Read the model definition and answer for the solid it produces. Units are mm, in the model's axes. Coordinates: 2 decimals unless noted, no trailing zeros. Write each loop counter-clockwise with the first axis right and the second up, starting at its lowest first coordinate (ties: lowest second). Pieces come first, ordered by that corner, then holes. Notation, with made-up numbers: (56, 53) -> (83, 53) arc R15 ccw to (83, 77) -> close; hole circle Ø5 at (4, -27). An arc over 180 degrees is marked (long way). Write item = value, one per line. Start each with the question number.
1) Flat-ended cylindrical pins translate along their axes: pin 1 Ø5.5 at (x, z) = (37, -100) entering from +Y; pin 2 Ø14 at (x, z) = (91.59, 59.68) entering from -Y; pin 3 Ø7 at (x, z) = (-77.5, 115) entering from -Y. Find the tip coordinate at first contact, or state that the pin passes through.
2) Section A-A (x = 0) is taken. Determine the outline of the cut face in (y, z), plus the area to 3 significant figures.
3) Section B-B (y = -6.5) is taken. Count the separate pieces of the cut face and the enclosed holes in it, plus the area to 3 significant figures.
4) Section C-C (x = 77.5) is taken. Determine the outline of the cut face in (y, z), plus the area to 3 significant figures.
5) Find the intervals of material crossed by line 1 along Z through (x, y) = (0, -3.5); line 2 along Z through (x, y) = (-76.2, -9.8); line 3 along Z through (x, y) = (42.5, -3.5), in increasing order. Write a range as from..to.
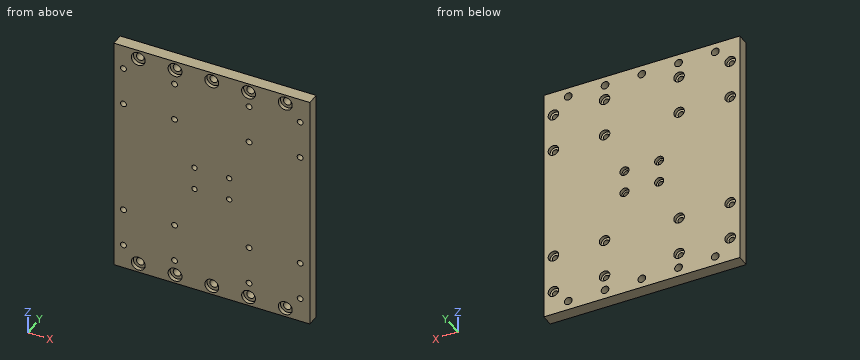
from build123d import *

# Parameters (mm, degrees)
F0_W      = 203.2
F0_H      = 249.9106
F0_R      = 3.048
F1_DEPTH  = 12.7
F2_R      = 2.794
F3_DEPTH  = 12.701
F4_R      = 4.0005
F5_DEPTH  = 12.701
F6_DEPTH  = 12.701
F7_R      = 7.1882
F8_DEPTH  = 4.064
F9_R      = 5.461
F9_R_2    = 4.699
F10_DEPTH = 3.81


with BuildPart() as f1:
    # F0 (on Front) → F1 (new body)
    with BuildSketch(Plane.XZ):
        Rectangle(F0_W, F0_H)
        with Locations((-91.5924, -99.5553)):
            Circle(F0_R, mode=Mode.SUBTRACT)
        with Locations((-38.6334, -99.5553)):
            Circle(F0_R, mode=Mode.SUBTRACT)
        with Locations((-91.5924, -59.6773)):
            Circle(F0_R, mode=Mode.SUBTRACT)
        with Locations((-38.6334, -59.6773)):
            Circle(F0_R, mode=Mode.SUBTRACT)
        with Locations((38.6334, -99.5553)):
            Circle(F0_R, mode=Mode.SUBTRACT)
        with Locations((91.5924, -99.5553)):
            Circle(F0_R, mode=Mode.SUBTRACT)
        with Locations((38.6334, -59.6773)):
            Circle(F0_R, mode=Mode.SUBTRACT)
        with Locations((91.5924, -59.6773)):
            Circle(F0_R, mode=Mode.SUBTRACT)
        with Locations((-91.5924, 59.6773)):
            Circle(F0_R, mode=Mode.SUBTRACT)
        with Locations((-38.6334, 59.6773)):
            Circle(F0_R, mode=Mode.SUBTRACT)
        with Locations((-91.5924, 99.5553)):
            Circle(F0_R, mode=Mode.SUBTRACT)
        with Locations((-38.6334, 99.5553)):
            Circle(F0_R, mode=Mode.SUBTRACT)
        with Locations((38.6334, 59.6773)):
            Circle(F0_R, mode=Mode.SUBTRACT)
        with Locations((91.5924, 59.6773)):
            Circle(F0_R, mode=Mode.SUBTRACT)
        with Locations((38.6334, 99.5553)):
            Circle(F0_R, mode=Mode.SUBTRACT)
        with Locations((91.5924, 99.5553)):
            Circle(F0_R, mode=Mode.SUBTRACT)
    extrude(amount=F1_DEPTH)

    # F2 (on face) → F3 (cut, through all)
    with BuildSketch(Plane.XZ.offset(12.7)):
        with Locations((-17.9959, 11.938)):
            Circle(F2_R)
        with Locations((17.9959, 11.938)):
            Circle(F2_R)
        with Locations((17.9959, -11.938)):
            Circle(F2_R)
        with Locations((-17.9959, -11.938)):
            Circle(F2_R)
    extrude(amount=-F3_DEPTH, mode=Mode.SUBTRACT)

    # F4 (on face) → F5 (cut, through all)
    with BuildSketch(Plane.XZ.offset(12.7)):
        with Locations((-76.2, 115.4303)):
            Circle(F4_R)
        with Locations((-38.1, 115.4303)):
            Circle(F4_R)
        with Locations((0, 115.4303)):
            Circle(F4_R)
        with Locations((38.1, 115.4303)):
            Circle(F4_R)
        with Locations((76.2, 115.4303)):
            Circle(F4_R)
        with Locations((-76.2, -115.4303)):
            Circle(F4_R)
        with Locations((-38.1, -115.4303)):
            Circle(F4_R)
        with Locations((0, -115.4303)):
            Circle(F4_R)
        with Locations((38.1, -115.4303)):
            Circle(F4_R)
        with Locations((76.2, -115.4303)):
            Circle(F4_R)
    extrude(amount=-F5_DEPTH, mode=Mode.SUBTRACT)

    # F2 (on face) → F6 (cut, through all)
    with BuildSketch(Plane.XZ.offset(12.7)):
        with Locations((-17.9959, 11.938)):
            Circle(F2_R)
        with Locations((17.9959, 11.938)):
            Circle(F2_R)
        with Locations((17.9959, -11.938)):
            Circle(F2_R)
        with Locations((-17.9959, -11.938)):
            Circle(F2_R)
    extrude(amount=-F6_DEPTH, mode=Mode.SUBTRACT)

    # F7 (on face) → F8 (cut)
    with BuildSketch(Plane.XZ.offset(12.7)):
        with Locations((0, -115.4303)):
            Circle(F7_R)
        with Locations((0, 115.4303)):
            Circle(F7_R)
        with Locations((-38.1, -115.4303)):
            Circle(F7_R)
        with Locations((-76.2, -115.4303)):
            Circle(F7_R)
        with Locations((38.1, -115.4303)):
            Circle(F7_R)
        with Locations((76.2, -115.4303)):
            Circle(F7_R)
        with Locations((-76.2, 115.4303)):
            Circle(F7_R)
        with Locations((-38.1, 115.4303)):
            Circle(F7_R)
        with Locations((38.1, 115.4303)):
            Circle(F7_R)
        with Locations((76.2, 115.4303)):
            Circle(F7_R)
    extrude(amount=-F8_DEPTH, mode=Mode.SUBTRACT)

    # F9 (on face) → F10 (cut)
    with BuildSketch(Plane(origin=(0, 0, 0), x_dir=(-1, 0, 0), z_dir=(0, 1, 0))):
        with Locations((-91.5924, 99.5553)):
            Circle(F9_R)
        with Locations((-38.6334, 99.5553)):
            Circle(F9_R)
        with Locations((38.6334, 99.5553)):
            Circle(F9_R)
        with Locations((91.5924, 99.5553)):
            Circle(F9_R)
        with Locations((-91.5924, 59.6773)):
            Circle(F9_R)
        with Locations((-38.6334, 59.6773)):
            Circle(F9_R)
        with Locations((38.6334, 59.6773)):
            Circle(F9_R)
        with Locations((91.5924, 59.6773)):
            Circle(F9_R)
        with Locations((-91.5924, -59.6773)):
            Circle(F9_R)
        with Locations((-38.6334, -59.6773)):
            Circle(F9_R)
        with Locations((38.6334, -59.6773)):
            Circle(F9_R)
        with Locations((91.5924, -59.6773)):
            Circle(F9_R)
        with Locations((91.5924, -99.5553)):
            Circle(F9_R)
        with Locations((38.6334, -99.5553)):
            Circle(F9_R)
        with Locations((-38.6334, -99.5553)):
            Circle(F9_R)
        with Locations((-91.5924, -99.5553)):
            Circle(F9_R)
        with Locations((-17.9959, 11.938)):
            Circle(F9_R_2)
        with Locations((17.9959, 11.938)):
            Circle(F9_R_2)
        with Locations((17.9959, -11.938)):
            Circle(F9_R_2)
        with Locations((-17.9959, -11.938)):
            Circle(F9_R_2)
    extrude(amount=-F10_DEPTH, mode=Mode.SUBTRACT)


solid = f1.part
Answer key:
q1.pin_1 = -3.81
q1.pin_2 = -12.7
q1.pin_3 = -8.64
q2.outline = (-12.7, -124.96) -> (0, -124.96) -> (0, -119.43) -> (-8.64, -119.43) -> (-8.64, -122.62) -> (-12.7, -122.62) -> close; (-12.7, -108.24) -> (-8.64, -108.24) -> (-8.64, -111.43) -> (0, -111.43) -> (0, 111.43) -> (-8.64, 111.43) -> (-8.64, 108.24) -> (-12.7, 108.24) -> close; (-12.7, 122.62) -> (-8.64, 122.62) -> (-8.64, 119.43) -> (0, 119.43) -> (0, 124.96) -> (-12.7, 124.96) -> close
q2.area = 2,920 mm^2
q3.separate_pieces = 1
q3.enclosed_holes = 30
q3.area = 49,700 mm^2
q4.outline = (-12.7, -124.96) -> (0, -124.96) -> (0, -119.21) -> (-8.64, -119.21) -> (-8.64, -122.5) -> (-12.7, -122.5) -> close; (-12.7, -108.36) -> (-8.64, -108.36) -> (-8.64, -111.65) -> (0, -111.65) -> (0, 111.65) -> (-8.64, 111.65) -> (-8.64, 108.36) -> (-12.7, 108.36) -> close; (-12.7, 122.5) -> (-8.64, 122.5) -> (-8.64, 119.21) -> (0, 119.21) -> (0, 124.96) -> (-12.7, 124.96) -> close
q4.area = 2,930 mm^2
q5.line_1 = -124.96..-119.43, -111.43..111.43, 119.43..124.96
q5.line_2 = -124.96..-122.62, -108.24..108.24, 122.62..124.96
q5.line_3 = -124.96..-103.41, -95.7..-63.53, -55.82..55.82, 63.53..95.7, 103.41..124.96
